Here's how the part is built. I have some questions about the finished solid (model axes, mm). A direction names the side the tool comes from. Round coordinates to 2 decimals unless told otherwise and drop trailing zeros. Loops run counter-clockwise (first coordinate to the right, second up) from the corner with the lowest first, then second, coordinate; pieces in that order, holes last. Notation, with made-up numbers: M -30,10.5 L -19,10.5 A24 ccw -19,43.5 Z; hole C 1,41 d3. An arc over 180 degrees is marked long. Put each result on its own line as item: value. Start each with the question number.
```python
from build123d import *

# Parameters (mm, degrees)
SKETCH_1_R          = 7
SKETCH_1_R_2        = 3.45
EXTRUDE_1_DEPTH     = 10
SKETCH_2_R          = 8.05
SKETCH_2_R_2        = 4
CUT_EXTRUDE_1_DEPTH = 8


with BuildPart() as part:
    # 草图1 → 凸台-拉伸1 (new body)
    with BuildSketch(Plane.XY):
        Polygon((-25, 0), (25, 0), (25, 26), (13, 26), (13, 85), (-13, 85), (-13, 26), (-25, 26), align=None)
        with Locations((0, 73)):
            Circle(SKETCH_1_R, mode=Mode.SUBTRACT)
        with Locations((-15, 13)):
            Circle(SKETCH_1_R_2, mode=Mode.SUBTRACT)
        with Locations((15, 13)):
            Circle(SKETCH_1_R_2, mode=Mode.SUBTRACT)
    extrude(amount=EXTRUDE_1_DEPTH)

    # 草图2 → 切除-拉伸1 (cut)
    with BuildSketch(Plane(origin=(0, 0, 0), x_dir=(-1, 0, 0), z_dir=(0, 0, -1))):
        with Locations((0, 73)):
            Circle(SKETCH_2_R)
        with Locations((0, 73)):
            Circle(SKETCH_2_R_2, mode=Mode.SUBTRACT)
    extrude(amount=-CUT_EXTRUDE_1_DEPTH, mode=Mode.SUBTRACT)


solid = part.part
```
1) Suppose I cut it at D-D (z = 4). Write out the boundary of the cut face in (x, y), plus the area to 3 significant figures.
2) If we mould it in two halves opening along Y, with no side actions, what happens to faces 5 (the face through (0, 0, 5)), 6 (the face through (-0.91, 79.94, 8.99)), 7 (the face through (-25, 13, 5))? For each: pulls with the +Y half, pulls with the -Y half, needs draft (parallel to the pull), parting line crosses it, or undercut.
3) Suppose I cut it at B-B (x = -15). Write out the boundary of the cut face in (y, z).
4) On a 3-axis mill with a long thin cutter (end or side, diameter ignored), from which of +Z, -Z, +X, -X, +Y, -Y can I reach the whole of each face in a straight line? I mean faces 1 (the face through (-19, 26, 5)), 2 (the face through (12.457, 15.332, 4.93)), 3 (the face through (19, 26, 5)), 4 (the face through (2, 80, 8)). Say none if no direction works.
5) I'm going to push flat-ended pins straight in: P1, Ø6, axis at y = 55.5, z = 2, coming from the -X side; P2, Ø12.5, axis at x = 0, y = 73, coming from the +Z side; P3, Ø8, axis at x = 3, y = 71, coming from the -Z side; P4, Ø5, axis at x = -16.5, z = 5.5, coming from the +Y side. Where does each tip first touch, or does it pass through?
6) Suppose I cut it at A-A (y = 13). Write out the boundary of the cut face in (x, z).
7) If I drill on probe 1 along X at (y, z) = (73, 8.65); probe 2 along Y at (x, z) = (0, 9.2); probe 3 along Y at (x, z) = (15, 7.75), over which ranges is the centre line in solid material (lowest first)? Write a range as from..to.
8) Suppose I cut it at C-C (y = 73). Write out the boundary of the cut face in (x, z), plus the area to 3 significant figures.
Results are:
1. outline: M -25,0 L 25,0 L 25,26 L 13,26 L 13,85 L -13,85 L -13,26 L -25,26 Z; hole C -15,13 d6.9; hole C 0,73 d16.1; hole C 15,13 d6.9
1. area: 2,560 mm²
2. face 5: pulls with the -Y half
2. face 6: undercut
2. face 7: needs draft
3. outline: M 0,0 L 9.55,0 L 9.55,10 L 0,10 Z; M 16.45,0 L 26,0 L 26,10 L 16.45,10 Z
4. face 1: +Z, -Z, -X, +Y
4. face 2: +Z, -Z
4. face 3: +Z, -Z, +X, +Y
4. face 4: -Z
5. P1: x = -13
5. P2: through
5. P3: z = 8
5. P4: y = 26
6. outline: M -25,0 L -18.45,0 L -18.45,10 L -25,10 Z; M -11.55,0 L 11.55,0 L 11.55,10 L -11.55,10 Z; M 18.45,0 L 25,0 L 25,10 L 18.45,10 Z
7. probe 1: -13..-7, 7..13
7. probe 2: 0..66, 80..85
7. probe 3: 0..9.55, 16.45..26
8. outline: M -13,0 L -8.05,0 L -8.05,8 L -7,8 L -7,10 L -13,10 Z; M 7,8 L 8.05,8 L 8.05,0 L 13,0 L 13,10 L 7,10 Z
8. area: 103 mm²
